Work out the finished part from the listing and answer in its coordinate system (mm). Coordinates: 2 decimals unless noted, no trailing zeros. Loops run counter-clockwise (first coordinate to the right, second up) from the corner with the lowest first, then second, coordinate; pieces in that order, holes last.
```python
from build123d import *

# Parameters (mm, degrees)
BLANKSKE_W              = 86
BLANKSKE_H              = 16.375
BLANK_DEPTH             = 6
TOOTHCUTSIM_DEPTH       = 88.750445156
TEETHCUTS_COUNT         = 21
TEETHCUTS_PITCH         = 4.319689894
ESQUISSE1_R             = 1.5
ENL_V_MAT_EXTRU_1_DEPTH = 88.750445156


with BuildPart() as part:
    # BlankSke → Blank (new body)
    with BuildSketch(Plane.XY):
        with Locations((43, 8.1875)):
            Rectangle(BLANKSKE_W, BLANKSKE_H)
    extrude(amount=-BLANK_DEPTH)

    # TooCutSkeSim → ToothCutSim (cut, through all)
    with BuildSketch(Plane.XY):
        Polygon((0.7824235, 13.28125), (-0.7824235, 13.28125), (-1.589090539, 16.4004), (1.589090539, 16.4004), align=None)
    toothcutsim = extrude(amount=-TOOTHCUTSIM_DEPTH, mode=Mode.SUBTRACT)

    # TeethCuts: ToothCutSim ×21
    with Locations(*[(i * TEETHCUTS_PITCH, 0, 0) for i in range(1, TEETHCUTS_COUNT)]):
        add(toothcutsim, mode=Mode.SUBTRACT)

    # Esquisse1 → Enlèv. mat.-Extru.1 (cut, through all)
    with BuildSketch(Plane.XY):
        with Locations((40, 5)):
            Circle(ESQUISSE1_R)
        with Locations((54, 5)):
            Circle(ESQUISSE1_R)
    extrude(amount=-ENL_V_MAT_EXTRU_1_DEPTH, mode=Mode.SUBTRACT)


solid = part.part
```
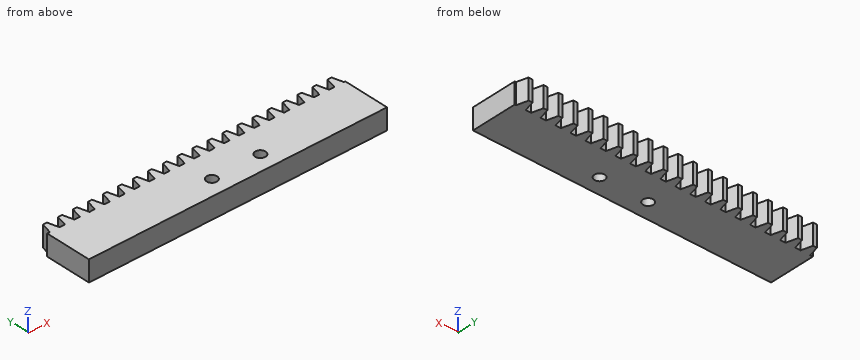
1. A cutting plane is placed at B-B, the plane z = -3.6. Count the separate pieces of the cut face and the enclosed holes in it, then the cut area to 3 significant figures.
2. This flat-tipped pin is pushed along its axis until it touches: P1, Ø0.5, axis at x = 60.5, z = -2.5, coming from the +Y side. Where does it stop, or does it pass through?
3. Straight lines are drawn through the part: probe 1 along Y at (x, z) = (54, -2.2) (3 decimals); probe 2 along X at (y, z) = (4.5, -3.45); probe 3 along X at (y, z) = (4, -4.85). For each, find the intervals that lie inside material, in ascending order.
4. A cutting plane is placed at A-A, the plane y = 5. Give the vertices of the cut face in (x, z).
Answers below:
1. separate pieces: 1
1. enclosed holes: 2
1. area: 1,250 mm2
2. P1: stops at y = 13.28
3. probe 1: y = 0 to 3.5, 6.5 to 16.375
3. probe 2: x = 0 to 38.59, 41.41 to 52.59, 55.41 to 86
3. probe 3: x = 0 to 38.88, 41.12 to 52.88, 55.12 to 86
4. outline: (0, -6) - (38.5, -6) - (38.5, 0) - (0, 0) - close; (41.5, -6) - (52.5, -6) - (52.5, 0) - (41.5, 0) - close; (55.5, -6) - (86, -6) - (86, 0) - (55.5, 0) - close
